```python
from build123d import *
from build123d.topology import SkipClean

# Parameters (mm, degrees)
SKETCH1_R                = 17.25
SKETCH1_R_2              = 12.25
BOSS_EXTRUDE1_DEPTH      = 4
SKETCH2_W                = 6
SKETCH2_H                = 6.066865377
CUT_EXTRUDE1_DEPTH       = 25.720942539
BOSS_EXTRUDE2_START      = -4
BOSS_EXTRUDE2_DEPTH      = 4
BOSS_EXTRUDE3_DEPTH      = 12.3
BOSS_EXTRUDE4_DEPTH      = 4
BOSS_EXTRUDE4_DEPTH_BACK = 4
SKETCH5_W                = 12.25
SKETCH5_H                = 26
CUT_EXTRUDE2_DEPTH       = 53.669881205
CUT_EXTRUDE2_DEPTH_BACK  = 53.669881205
SKETCH6_R                = 1.7
SKETCH7_R                = 3.05
CUT_EXTRUDE6_DEPTH       = 4
CHAMFER1_SIZE            = 4
BOSS_EXTRUDE5_REACH      = 55.745
BOSS_EXTRUDE6_DEPTH      = 6
BOSS_EXTRUDE6_DEPTH_BACK = 16.3
SKETCH9_W                = 4
SKETCH9_H                = 13.772279307
BOSS_EXTRUDE7_DEPTH      = 4
BOSS_EXTRUDE8_DEPTH      = 16.3
SKETCH12_W               = 4
SKETCH12_H               = 15
BOSS_EXTRUDE9_DEPTH      = 22.3
CHAMFER2_START           = 13.712068893
CHAMFER2_OUTLINE_W       = 11
CHAMFER2_OUTLINE_H       = 13
CHAMFER2_DEPTH           = 5.287931107
CHAMFER3_START           = 14.289419162
CHAMFER3_OUTLINE_W       = 10
CHAMFER3_OUTLINE_H       = 11
CHAMFER3_DEPTH           = 10.664231106
BOSS_EXTRUDE10_DEPTH     = 3
BOSS_EXTRUDE11_DEPTH     = 4


with BuildPart() as part:
    # Sketch1 → Boss-Extrude1 (new body)
    with BuildSketch(Plane(origin=(0, 0, 0), x_dir=(1, 0, 0), z_dir=(0, 1, 0))):
        with Locations(Location((0, 0, 0), (0, 0, 270))):
            Circle(SKETCH1_R)
        with Locations(Location((0, 0, 0), (0, 0, 270))):
            Circle(SKETCH1_R_2, mode=Mode.SUBTRACT)
    extrude(amount=BOSS_EXTRUDE1_DEPTH)

    # Sketch2 → Cut-Extrude1 (cut, through all)
    with BuildSketch(Plane(origin=(0, 4, 0), x_dir=(1, 0, 0), z_dir=(0, 1, 0))):
        with Locations((-2, -14.216567312)):
            Rectangle(SKETCH2_W, SKETCH2_H)
    extrude(amount=-CUT_EXTRUDE1_DEPTH, mode=Mode.SUBTRACT)

    # Sketch3 → Boss-Extrude2 (add)
    with BuildSketch(Plane(origin=(0, 4, 0), x_dir=(1, 0, 0), z_dir=(0, 1, 0)).offset(BOSS_EXTRUDE2_START)):
        with BuildLine():
            Line((-5, -16.509466981), (-5, -22.220990099))
            Line((-5, -22.220990099), (-17.25, -22.220990099))
            Line((-17.25, -22.220990099), (-17.25, 0))
            ThreePointArc((-17.25, 0), (-13.853023136, -10.278922609), (-5, -16.509466981))
        make_face()
    extrude(amount=BOSS_EXTRUDE2_DEPTH)

    # Sketch4 → Boss-Extrude3 (add)
    with SkipClean():  # the faces are left unmerged after this step: merging them gives an invalid solid
        with BuildSketch(Plane(origin=(0, 4, 0), x_dir=(1, 0, 0), z_dir=(0, 1, 0))):
            with BuildLine():
                Line((-17.25, 0), (-17.25, -7.145183951))
                Line((-17.25, -7.145183951), (-11.317524273, -4.687872046))
                ThreePointArc((-11.317524273, -4.687872046), (-12.25, 0), (-11.317524273, 4.687872046))
                Line((-11.317524273, 4.687872046), (-15.936921936, 6.601289208))
                ThreePointArc((-15.936921936, 6.601289208), (-16.918546087, 3.365308055), (-17.25, 0))
            make_face()
            with BuildLine():
                Line((10.608811196, 6.125), (14.938938215, 8.625))
                ThreePointArc((14.938938215, 8.625), (17.25, 0), (14.938938215, -8.625))
                Line((14.938938215, -8.625), (10.608811196, -6.125))
                ThreePointArc((10.608811196, -6.125), (12.25, 0), (10.608811196, 6.125))
            make_face()
        extrude(amount=BOSS_EXTRUDE3_DEPTH)

    # Sketch5 → Boss-Extrude4 (add, two sides: drawn at the far end of the back side and taken through both)
    with SkipClean():  # the faces are left unmerged after this step: merging them gives an invalid solid
        with BuildSketch(Plane(origin=(0, 4, 0), x_dir=(1, 0, 0), z_dir=(0, 1, 0)).offset(-BOSS_EXTRUDE4_DEPTH_BACK)):
            with Locations((-11.125, -35.220990099)):
                Rectangle(SKETCH5_W, SKETCH5_H)
        extrude(amount=BOSS_EXTRUDE4_DEPTH + BOSS_EXTRUDE4_DEPTH_BACK)

    # Sketch6 → Cut-Extrude2 (cut, two sides: drawn at the far end of the back side and taken through both)
    with SkipClean():  # the faces are left unmerged after this step: merging them gives an invalid solid
        with BuildSketch(Plane(origin=(0, 4, 0), x_dir=(1, 0, 0), z_dir=(0, 1, 0)).offset(-CUT_EXTRUDE2_DEPTH_BACK)):
            with Locations(Location((-13.25, -43.720990099, 0), (0, 0, 270))):
                Circle(SKETCH6_R)
            with Locations(Location((-13.25, -35.220990099, 0), (0, 0, 270))):
                Circle(SKETCH6_R)
            with Locations(Location((-13.25, -26.720990099, 0), (0, 0, 270))):
                Circle(SKETCH6_R)
        extrude(amount=CUT_EXTRUDE2_DEPTH + CUT_EXTRUDE2_DEPTH_BACK, mode=Mode.SUBTRACT)

    # Sketch7 → Cut-Extrude6 (cut)
    with SkipClean():  # the faces are left unmerged after this step: merging them gives an invalid solid
        with BuildSketch(Plane.XZ):
            with Locations(Location((-13.25, 43.720990099, 0), (0, 0, 270))):
                Circle(SKETCH7_R)
            with Locations(Location((-13.25, 35.220990099, 0), (0, 0, 270))):
                Circle(SKETCH7_R)
            with Locations(Location((-13.25, 26.720990099, 0), (0, 0, 270))):
                Circle(SKETCH7_R)
        extrude(amount=-CUT_EXTRUDE6_DEPTH, mode=Mode.SUBTRACT)

    # Chamfer1
    chamfer1_edges = [part.edges().sort_by_distance(p)[0] for p in [
        (-11.125, 4, 22.220990099),
    ]]
    chamfer(chamfer1_edges, length=CHAMFER1_SIZE - 0.0001)  # a hair under: the kernel refuses the full size

    # Boss-Extrude5: up to this face of the body (flat: up to its plane)
    boss_extrude5_end = Plane(part.part.faces().sort_by_distance((-14.634101331, 16.3, 0.270569761))[0])
    # Sketch8 → Boss-Extrude5 (add, up to the picked face)
    with BuildSketch(Plane.XZ, mode=Mode.PRIVATE) as boss_extrude5_sk1:
        with BuildLine():
            Line((-17.25, 0), (-17.25, 7.170990099))
            Line((-17.25, 7.170990099), (-19.25, 7.170990099))
            Line((-19.25, 7.170990099), (-19.25, -6.601289208))
            Line((-19.25, -6.601289208), (-15.936921936, -6.601289208))
            ThreePointArc((-15.936921936, -6.601289208), (-16.918546087, -3.365308055), (-17.25, 0))
        make_face()
    boss_extrude5_tool1 = split(extrude(boss_extrude5_sk1.sketch, amount=-BOSS_EXTRUDE5_REACH, mode=Mode.PRIVATE), bisect_by=boss_extrude5_end, keep=Keep.BOTH, mode=Mode.PRIVATE)
    add(boss_extrude5_tool1.solids().sort_by(Axis((-18.119805, 0, -0.206337), (0, 1, 0)))[0])

    # Sketch9 → Boss-Extrude6 (add, two sides: drawn at the far end of the back side and taken through both)
    with BuildSketch(Plane(origin=(0, 16.3, 0), x_dir=(1, 0, 0), z_dir=(0, 1, 0)).offset(-BOSS_EXTRUDE6_DEPTH_BACK)):
        with Locations((-21.25, -0.284850446)):
            Rectangle(SKETCH9_W, SKETCH9_H)
    extrude(amount=BOSS_EXTRUDE6_DEPTH + BOSS_EXTRUDE6_DEPTH_BACK)

    # Sketch10 → Boss-Extrude7 (add)
    with BuildSketch(Plane.XZ):
        with BuildLine():
            Line((-5, 24.220990099), (1, 24.220990099))
            Line((1, 24.220990099), (1, 17.220990099))
            ThreePointArc((1, 17.220990099), (3.021020736, 16.983401712), (5, 16.509466981))
            Line((5, 16.509466981), (5, 26.220990099))
            ThreePointArc((5, 26.220990099), (4.414213562, 27.635203662), (3, 28.220990099))
            Line((3, 28.220990099), (-5, 28.220990099))
            Line((-5, 28.220990099), (-5, 24.220990099))
        make_face()
    extrude(amount=-BOSS_EXTRUDE7_DEPTH)

    # Sketch11 → Boss-Extrude8 (add)
    with BuildSketch(Plane.XZ):
        with BuildLine():
            Line((15.534236383, 7.5), (19.25, 7.5))
            Line((19.25, 7.5), (19.25, -7.5))
            Line((19.25, -7.5), (15.534236383, -7.5))
            ThreePointArc((15.534236383, -7.5), (17.25, 0), (15.534236383, 7.5))
        make_face()
    extrude(amount=-BOSS_EXTRUDE8_DEPTH)

    # Sketch12 → Boss-Extrude9 (add)
    with BuildSketch(Plane.XZ):
        with Locations((21.25, 0)):
            Rectangle(SKETCH12_W, SKETCH12_H)
    extrude(amount=-BOSS_EXTRUDE9_DEPTH)

    # Chamfer2: read off the stored shape, not the designer's step
    # Chamfer2 outline → Chamfer2 (cut)
    with BuildSketch(Plane(origin=(0, 0, 0), x_dir=(0.8164965809277258, 0.40824829046386313, 0.40824829046386313), z_dir=(0.5773502691896258, -0.5773502691896258, -0.5773502691896258)).offset(CHAMFER2_START)):
        with Locations((14.5, -5.5)):
            Rectangle(CHAMFER2_OUTLINE_W, CHAMFER2_OUTLINE_H)
    extrude(amount=CHAMFER2_DEPTH, mode=Mode.SUBTRACT)

    # Chamfer3: read off the stored shape, not the designer's step
    # Chamfer3 outline → Chamfer3 (cut)
    with BuildSketch(Plane(origin=(0, 0, 0), x_dir=(0.8164965809277258, 0.40824829046386313, -0.40824829046386313), z_dir=(0.5773502691896258, -0.5773502691896258, 0.5773502691896258)).offset(CHAMFER3_START)):
        with Locations((15, 5.5)):
            Rectangle(CHAMFER3_OUTLINE_W, CHAMFER3_OUTLINE_H)
    extrude(amount=CHAMFER3_DEPTH, mode=Mode.SUBTRACT)

    # Sketch13 → Boss-Extrude10 (add)
    with BuildSketch(Plane(origin=(0, 4, 0), x_dir=(1, 0, 0), z_dir=(0, 1, 0))):
        with BuildLine():
            Line((-15.936921936, 6.601289208), (-11.317524273, 4.687872046))
            ThreePointArc((-11.317524273, 4.687872046), (-0.801188333, 12.22377181), (10.608811196, 6.125))
            Line((10.608811196, 6.125), (14.938938215, 8.625))
            ThreePointArc((14.938938215, 8.625), (-1.128203979, 17.213066426), (-15.936921936, 6.601289208))
        make_face()
    extrude(amount=BOSS_EXTRUDE10_DEPTH)

    # Sketch14 → Boss-Extrude11 (add)
    with BuildSketch(Plane(origin=(0, 4, 0), x_dir=(1, 0, 0), z_dir=(0, 1, 0))):
        with BuildLine():
            Line((14.938938215, -8.625), (10.608811196, -6.125))
            ThreePointArc((10.608811196, -6.125), (6.553261748, -10.349746879), (1, -12.209115447))
            Line((1, -12.209115447), (1, -24.220990099))
            Line((1, -24.220990099), (-5, -24.220990099))
            Line((-5, -24.220990099), (-5, -28.220990099))
            Line((-5, -28.220990099), (3, -28.220990099))
            ThreePointArc((3, -28.220990099), (4.414213562, -27.635203662), (5, -26.220990099))
            Line((5, -26.220990099), (5, -16.509466981))
            ThreePointArc((5, -16.509466981), (10.720611885, -13.514103034), (14.938938215, -8.625))
        make_face()
    extrude(amount=BOSS_EXTRUDE11_DEPTH)


solid = part.part
```
The listing builds one solid part. Answer for the finished solid, in the listing's coordinates (mm). A direction names the side the tool comes from. Give positions to 0.01 mm unless a question says otherwise; leave off trailing zeros. Order: outer loops, then holes, each group sorted by start corner. A loop starts at its lowest first (then second) coordinate and runs counter-clockwise, first axis right, second up. Notation, with made-up numbers: (88, 44.25) -> (117, 44.25) arc R16 cw to (117, 74.25) -> close; hole circle Ø5 at (35.25, 28.25). An arc over 180 degrees is marked (long way). One line per item, written item: value.
1) A tool of negligible diameter and unlimited length cuts with its end or side. For faces 1 (the cylindrical face through (-13.12, 1.97, 38.27)), 2 (the flat face through (-13.59, 11.58, -5.63)), 3 (the flat face through (-14.325, 10.064, 5.934)), from which of +Z, -Z, +X, -X, +Y, -Y can it reach the whole face along a straight path? Write none if from no direction.
Reported:
face 1: -Y
face 2: -Z, +Y
face 3: +Y
2) Determine the mould class of faces 4 (the flat face through (-19.25, 19, 0)), 5 (the flat face through (23.25, 13, 0)), 6 (the flat face through (-5.5, 0, 15.9)) for opening direction X: pulls with the +X half, pulls with the -X half, needs draft (parallel to the pull), parting line crosses it, or undercut.
Reported:
face 4: undercut
face 5: pulls with the +X half
face 6: needs draft
3) Flat-ended cylindrical pins translate along their axes: P1, Ø4, axis at y = 2.5, z = 19, coming from the +X side; P2, Ø10, axis at y = 12.5, z = 28, coming from the -X side; P3, Ø5, axis at x = 2, z = 15.5, coming from the +Y side; P4, Ø10, axis at y = 17.5, z = 17, coming from the -X side. Find the tip coordinate at first contact, or state that the pin passes through.
Reported:
P1: stops at x = 5
P2: stops at x = -17.25
P3: stops at y = 8
P4: passes through
4) Find section C-C, the plane y = 3.25. Determine the outline of the cut face in (x, z).
Reported:
outline: (-23.25, -6.6) -> (-15.94, -6.6) arc R17.25 ccw to (15.53, -7.5) -> (19.5, -7.5) -> (23.25, -3.75) -> (23.25, 4.75) -> (20.5, 7.5) -> (15.53, 7.5) arc R17.25 ccw to (5, 16.51) -> (5, 26.22) arc R2 ccw to (3, 28.22) -> (-5, 28.22) -> (-5, 48.22) -> (-17.25, 48.22) -> (-17.25, 7.17) -> (-23.25, 7.17) -> close; hole circle Ø6.1 at (-13.25, 26.72); hole circle Ø6.1 at (-13.25, 35.22); hole circle Ø6.1 at (-13.25, 43.72); hole (-5, 11.18) arc R12.25 ccw (long way) to (1, 12.21) -> (1, 24.22) -> (-5, 24.22) -> close
5) Find section D-D, the plane z = 3. Determine the outline of the cut face in (x, y).
Reported:
outline: (-23.25, 0) -> (-11.88, 0) -> (-11.88, 16.3) -> (-19.25, 16.3) -> (-19.25, 22.3) -> (-23.25, 22.3) -> close; (11.88, 0) -> (21.75, 0) -> (23.25, 1.5) -> (23.25, 22.3) -> (19.25, 22.3) -> (19.25, 16.3) -> (11.88, 16.3) -> close
6) Find section A-A, the plane y = 15.25. Determine the outline of the cut face in (x, z) (3 decimals), plus the area to 3 significant figures.
Reported:
outline: (-23.25, -6.601) -> (-15.937, -6.601) -> (-11.318, -4.688) arc R12.25 cw to (-11.318, 4.688) -> (-17.25, 7.145) -> (-17.25, 7.171) -> (-23.25, 7.171) -> close; (10.609, -6.125) -> (14.939, -8.625) arc R17.25 ccw to (15.534, -7.5) -> (23.25, -7.5) -> (23.25, 7.5) -> (15.534, 7.5) arc R17.25 ccw to (14.939, 8.625) -> (10.609, 6.125) arc R12.25 cw to start
area: 322 mm^2
7) Find the intervals of material crossed by line 1 (Z direction, x = -13.25, y = 5.35); line 2 (Z direction, x = -13.25, y = 5.05); line 3 (Z direction, x = 0.5, y = 3.25), in increasing order.
Reported:
line 1: z = -11.05 to 5.49, 19.57 to 25.02, 28.42 to 33.52, 36.92 to 42.02, 45.42 to 48.22
line 2: z = -11.05 to 5.49, 19.27 to 25.02, 28.42 to 33.52, 36.92 to 42.02, 45.42 to 48.22
line 3: z = -17.24 to -12.24, 24.22 to 28.22
8) Find section B-B, the plane x = 0. Determine the outline of the cut face in (y, z), plus the area to 3 significant figures.
Reported:
outline: (0, -17.25) -> (7, -17.25) -> (7, -12.25) -> (0, -12.25) -> close; (0, 24.22) -> (8, 24.22) -> (8, 28.22) -> (0, 28.22) -> close
area: 67.0 mm^2
